```python
from build123d import *

# Parameters (mm, degrees)
EXTRUDE_1_DEPTH     = 2.1
SKETCH_3_R          = 3.3
SKETCH_3_R_2        = 2.25
EXTRUDE_2_DEPTH     = 2.7
SKETCH_5_R          = 1.2
CUT_EXTRUDE_1_DEPTH = 2.7


with BuildPart() as part:
    # 草图2 → 凸台-拉伸1 (new body)
    with BuildSketch(Plane(origin=(0, 0, 0), x_dir=(1, 0, 0), z_dir=(0, 1, 0))):
        with BuildLine():
            Line((-16.16625, 1.892712587), (-0.28875, 3.287342914))
            ThreePointArc((-0.28875, 3.287342914), (3.3, 0), (-0.28875, -3.287342914))
            Line((-0.28875, -3.287342914), (-16.16625, -1.892712587))
            ThreePointArc((-16.16625, -1.892712587), (-17.9, 0), (-16.16625, 1.892712587))
        make_face()
    extrude(amount=EXTRUDE_1_DEPTH)

    # 草图3 → 凸台-拉伸2 (add)
    with BuildSketch(Plane(origin=(0, 2.1, 0), x_dir=(1, 0, 0), z_dir=(0, 1, 0))):
        with Locations(Location((0, 0, 0), (0, 0, 95.019800132))):
            Circle(SKETCH_3_R)
        with Locations(Location((0, 0, 0), (0, 0, 90))):
            Circle(SKETCH_3_R_2, mode=Mode.SUBTRACT)
    extrude(amount=EXTRUDE_2_DEPTH)

    # 草图5 → 切除-拉伸1 (cut)
    with BuildSketch(Plane(origin=(0, 2.1, 0), x_dir=(1, 0, 0), z_dir=(0, 1, 0))):
        with Locations(Location((0, 0, 0), (0, 0, 270))):
            Circle(SKETCH_5_R)
    extrude(amount=-CUT_EXTRUDE_1_DEPTH, mode=Mode.SUBTRACT)


solid = part.part
```
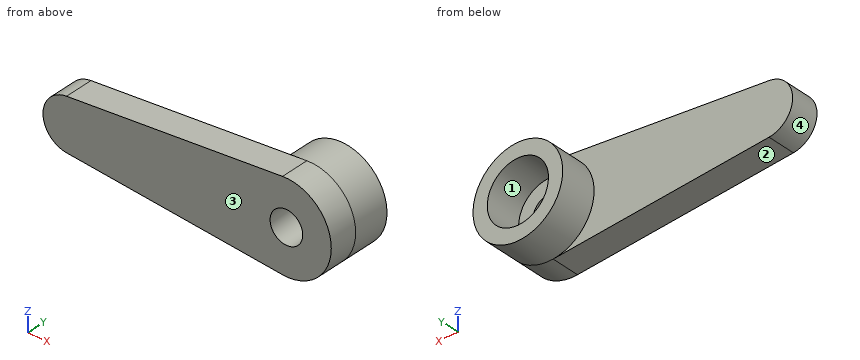
Work out the finished part from the listing and answer in its coordinate system (mm). Face numbers are marked on the shaded views. Give positions to 0.01 mm unless a question says otherwise; leave off trailing zeros. Write each loop counter-clockwise with the first axis right and the second up, starting at its lowest first coordinate (ties: lowest second). Pieces come first, ordered by that corner, then holes. Notation, with made-up numbers: (-36, 19) - (14, 19) arc R19 ccw to (14, 37) - close; hole circle Ø7 at (-36.75, -36.5). An arc over 180 degrees is marked (long way). Use one line per item in the form item = value.
1. Each of these flat-tipped pins is pushed along its axis until it touches: pin 1 Ø2 at (x, y) = (-14, 3) entering from -Z; pin 2 Ø1.5 at (y, z) = (2.5, 2) entering from +X; pin 3 Ø2 at (x, z) = (-1, -0.5) entering from +Y. Where does it stop, or does it pass through?
Filled in:
pin_1 = -2.12
pin_2 = 3.05
pin_3 = 2.1
2. A cutting plane is placed at C-C (y = 1.15). Write down the section's boundary in (x, z), and give its area (3 significant figures).
Filled in:
outline = (-16.17, -1.89) - (-0.29, -3.29) arc R3.3 ccw (long way) to (-0.29, 3.29) - (-16.17, 1.89) arc R1.9 ccw to start; hole circle Ø2.4 at (0, 0)
area = 102 mm^2
3. A cutting plane is placed at A-A (x = 0). Write down the section's boundary in (y, z).
Filled in:
outline = (0, -3.3) - (4.8, -3.3) - (4.8, -2.25) - (2.1, -2.25) - (2.1, -1.2) - (0, -1.2) - close; (0, 1.2) - (2.1, 1.2) - (2.1, 2.25) - (4.8, 2.25) - (4.8, 3.3) - (0, 3.3) - close
4. Consider L1, parallel to X at y = 3.6, z = 0; L2, parallel to X at y = 1.4, z = 0; L3, parallel to Y at x = -6.25, z = -0.5. Determine where each line is inside the solid, lowest interval first.
Filled in:
L1 = -3.3 to -2.25, 2.25 to 3.3
L2 = -17.9 to -1.2, 1.2 to 3.3
L3 = 0 to 2.1
5. A cutting plane is placed at B-B (z = 0.25). Write down the section's boundary in (x, y).
Filled in:
outline = (-17.88, 0) - (-1.17, 0) - (-1.17, 2.1) - (-2.24, 2.1) - (-2.24, 4.8) - (-3.29, 4.8) - (-3.29, 2.1) - (-17.88, 2.1) - close; (1.17, 0) - (3.29, 0) - (3.29, 4.8) - (2.24, 4.8) - (2.24, 2.1) - (1.17, 2.1) - close
6. A cutting plane is placed at D-D (z = -2.5). Write down the section's boundary in (x, y), and give its area (3 significant figures).
Filled in:
outline = (-9.25, 0) - (2.15, 0) - (2.15, 4.8) - (-2.15, 4.8) - (-2.15, 2.1) - (-9.25, 2.1) - close
area = 35.6 mm^2
7. Determine the mould class of the marked faces 1, 2, 3 and 4 for opening direction Z: released by +Z, released by -Z, zero draft, split by the parting line, or undercut.
Filled in:
face_1 = undercut
face_2 = released by -Z
face_3 = zero draft
face_4 = split by the parting line
